Here's how the part is built. I have some questions about the finished solid (model axes, mm). Give positions to 0.01 mm unless a question says otherwise; leave off trailing zeros. Order: outer loops, then holes, each group sorted by start corner. A loop starts at its lowest first (then second) coordinate and runs counter-clockwise, first axis right, second up. Notation, with made-up numbers: M 86,40 L 137,40 A26 ccw 137,62 Z; hole C 58.25,21 d8. An arc over 180 degrees is marked long. One line per item, written item: value. Start each with the question number.
from build123d import *

# Parameters (mm, degrees)
BOSS_EXTRUDE1_START = -63
BOSS_EXTRUDE1_DEPTH = 1.6
CHAMFER1_SIZE       = 0.3
BOSS_EXTRUDE2_START = 61.3
SKETCH2_W           = 1
SKETCH2_H           = 6
BOSS_EXTRUDE2_DEPTH = 0.31
BOSS_EXTRUDE3_START = 73.19
SKETCH3_W           = 1
SKETCH3_H           = 6
BOSS_EXTRUDE3_DEPTH = 0.31
BOSS_EXTRUDE4_START = 65.9
SKETCH4_W           = 0.7
SKETCH4_H           = 1.3
BOSS_EXTRUDE4_DEPTH = 3


with BuildPart() as part:
    # Sketch1 → Boss-Extrude1 (new body)
    with BuildSketch(Plane(origin=(0, 0, 0), x_dir=(0, 0, -1), z_dir=(1, 0, 0)).offset(BOSS_EXTRUDE1_START)):
        with BuildLine():
            Line((-73.2, 110), (-73.2, 116))
            ThreePointArc((-73.2, 116), (-71.501219331, 120.101219331), (-67.4, 121.8))
            ThreePointArc((-67.4, 121.8), (-63.298780669, 120.101219331), (-61.6, 116))
            Line((-61.6, 116), (-61.6, 110))
            ThreePointArc((-61.6, 110), (-63.298780669, 105.898780669), (-67.4, 104.2))
            ThreePointArc((-67.4, 104.2), (-71.501219331, 105.898780669), (-73.2, 110))
        make_face()
    extrude(amount=BOSS_EXTRUDE1_DEPTH)

    # Chamfer1
    chamfer1_edges = [part.edges().sort_by_distance(p)[0] for p in [
        (-63, 104.2, 67.4),
        (-63, 113, 73.2),
        (-63, 121.8, 67.4),
        (-63, 113, 61.6),
    ]]
    chamfer(chamfer1_edges, length=CHAMFER1_SIZE)

    # Sketch2 → Boss-Extrude2 (add)
    with BuildSketch(Plane.XY.offset(BOSS_EXTRUDE2_START)):
        with Locations((-62.2, 113)):
            Rectangle(SKETCH2_W, SKETCH2_H)
    extrude(amount=BOSS_EXTRUDE2_DEPTH)

    # Sketch3 → Boss-Extrude3 (add)
    with BuildSketch(Plane.XY.offset(BOSS_EXTRUDE3_START)):
        with Locations((-62.2, 113)):
            Rectangle(SKETCH3_W, SKETCH3_H)
    extrude(amount=BOSS_EXTRUDE3_DEPTH)


with BuildPart() as body_2:
    # Sketch4 → Boss-Extrude4 (new body)
    with BuildSketch(Plane.XY.offset(BOSS_EXTRUDE4_START)):
        with Locations((-62.75, 104.75)):
            Rectangle(SKETCH4_W, SKETCH4_H)
    extrude(amount=BOSS_EXTRUDE4_DEPTH)


with BuildPart() as part_1:
    add(part.part)

    # Combine1: cut body 2
    add(body_2.part, mode=Mode.SUBTRACT)


solid = part_1.part
Item 1: I want a section at A-A on y = 114.75. Write out the boundary of the cut face in (x, z).
Item 2: Will these pins go through, and if not, where does the flat tip stop? P1, Ø0.7, axis at x = -62.5, y = 105, coming from the +Z side; P2, Ø0.5, axis at x = -62.5, y = 105, coming from the -Z side.
Item 3: We'd pull the mould along Z, two halves only. Please class faces 1 (the face through (-62.4, 105, 67)), 2 (the face through (-63, 113, 67)), 3 (the face through (-62.885, 106.541, 71.822)), 4 (the face through (-62.885, 106.623, 62.915)): +Z half, -Z half, draft (parallel to the pull), parting line (faces both ways), or undercut.
Item 4: I want a section at B-B on x = -61.95. Write out the boundary of the cut face in (y, z).
Item 5: Please list where these lines run through material, in increasing order: probe 1 along Z at (x, y) = (-62.9, 116); probe 2 along Y at (x, z) = (-62, 71); probe 3 along Z at (x, y) = (-61.8, 120.75). Write a range as [from, to].
Answer below:
1. outline: M -63,61.9 L -62.7,61.6 L -62.7,61.3 L -61.7,61.3 L -61.7,61.6 L -61.4,61.6 L -61.4,73.2 L -61.7,73.2 L -61.7,73.5 L -62.7,73.5 L -62.7,73.2 L -63,72.9 Z
2. P1: stops at z = 70.87
2. P2: stops at z = 64.07
3. face 1: undercut
3. face 2: draft
3. face 3: +Z half
3. face 4: -Z half
4. outline: M 110,61.3 L 116,61.3 L 116,61.6 A5.8 ccw 116,73.2 L 116,73.5 L 110,73.5 L 110,73.2 A5.8 ccw 110,61.6 Z
5. probe 1: z = [61.8, 73]
5. probe 2: y = [105.45, 120.55]
5. probe 3: z = [64.07, 70.73]
